Study the drawing (mm; zero at the part's minimum x, y, z) and answer. Coordinates: 2 decimals unless noted, no trailing zeros. Order: outer loops, then holes, each group sorted by start corner. A loop starts at its lowest first (then second) coordinate and runs counter-clockwise, first axis right, second up.
1. Find the intervals of material crossed by probe 1 along Z at (x, y) = (51, 1.1); probe 2 along Z at (x, y) = (74, 0.4); probe 3 along X at (y, z) = (0.4, 15) (1 decimal), in increasing order.
2. The part is cut by section A-A, the plane z = 29. Give the vertices of the cut face in (x, y).
3. The part is cut by section B-B, the plane y = 1. Give the vertices of the cut face in (x, z).
4. The part is cut by section C-C, the plane x = 48. Give the vertices of the cut face in (y, z), then the cut area to 3 significant figures.
5. The part is cut by section D-D, the plane z = 13. Give the vertices of the cut face in (x, y).
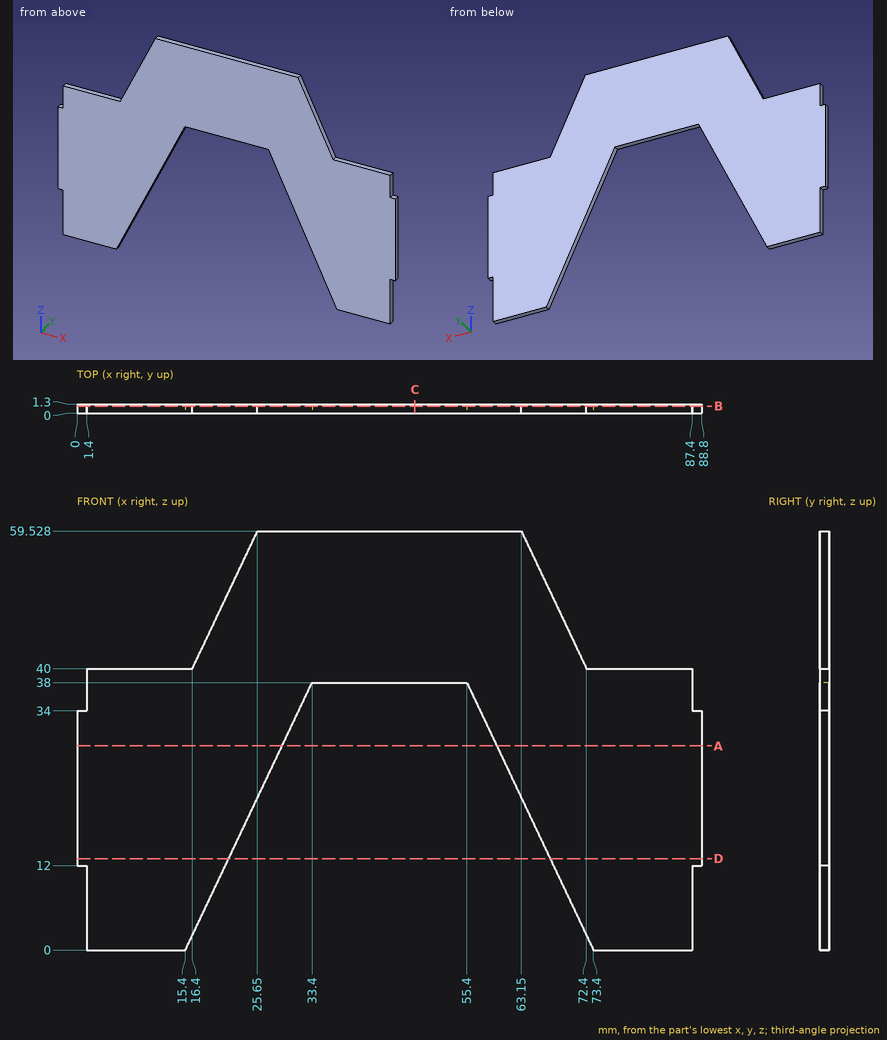
Geometry says:
1. probe 1: z = 38 to 59.53
1. probe 2: z = 0 to 40
1. probe 3: x = 0 to 22.5, 66.3 to 88.8
2. outline: (0, 0) - (29.14, 0) - (29.14, 1.3) - (0, 1.3) - close; (59.66, 0) - (88.8, 0) - (88.8, 1.3) - (59.66, 1.3) - close
3. outline: (0, 12) - (1.4, 12) - (1.4, 0) - (15.4, 0) - (33.4, 38) - (55.4, 38) - (73.4, 0) - (87.4, 0) - (87.4, 12) - (88.8, 12) - (88.8, 34) - (87.4, 34) - (87.4, 40) - (72.4, 40) - (63.15, 59.53) - (25.65, 59.53) - (16.4, 40) - (1.4, 40) - (1.4, 34) - (0, 34) - close
4. outline: (0, 38) - (1.3, 38) - (1.3, 59.53) - (0, 59.53) - close
4. area: 28.0 mm2
5. outline: (0, 0) - (21.56, 0) - (21.56, 1.3) - (0, 1.3) - close; (67.24, 0) - (88.8, 0) - (88.8, 1.3) - (67.24, 1.3) - close
